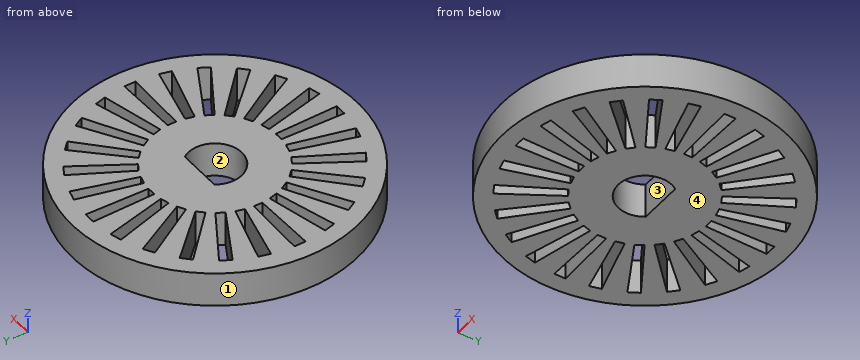
from build123d import *

# Parameters (mm, degrees)
CROQUIS1_R              = 12.84605
SALIENTE_EXTRUIR2_DEPTH = 3.1242


with BuildPart() as part:
    # Croquis1 → Saliente-Extruir2 (new body)
    with BuildSketch(Plane.XY):
        Circle(CROQUIS1_R)
        Polygon((0.508, 11.32205), (0.381, 5.73405), (-0.381, 5.73405), (-0.508, 11.32205), align=None, mode=Mode.SUBTRACT)
        Polygon((-7.646688087, -8.365108577), (-8.365108577, -7.646688087), (-4.323993322, -3.785177955), (-3.785177955, -4.323993322), align=None, mode=Mode.SUBTRACT)
        Polygon((-5.221084095, -10.059182923), (-6.100965905, -9.551182923), (-3.196980679, -4.775332967), (-2.537069321, -5.156332967), align=None, mode=Mode.SUBTRACT)
        Polygon((-2.43967185, -11.067740576), (-3.421052489, -10.804780427), (-1.852099085, -5.440056928), (-1.116063606, -5.63727704), align=None, mode=Mode.SUBTRACT)
        Polygon((-9.551182923, -6.100965905), (-10.059182923, -5.221084095), (-5.156332967, -2.537069321), (-4.775332967, -3.196980679), align=None, mode=Mode.SUBTRACT)
        Polygon((-11.32205, -0.508), (-11.32205, 0.508), (-5.73405, 0.381), (-5.73405, -0.381), align=None, mode=Mode.SUBTRACT)
        Polygon((-10.804780427, -3.421052489), (-11.067740576, -2.43967185), (-5.63727704, -1.116063606), (-5.440056928, -1.852099085), align=None, mode=Mode.SUBTRACT)
        Polygon((0.508, -11.32205), (-0.508, -11.32205), (-0.381, -5.73405), (0.381, -5.73405), align=None, mode=Mode.SUBTRACT)
        Polygon((3.421052489, -10.804780427), (2.43967185, -11.067740576), (1.116063606, -5.63727704), (1.852099085, -5.440056928), align=None, mode=Mode.SUBTRACT)
        Polygon((6.100965905, -9.551182923), (5.221084095, -10.059182923), (2.537069321, -5.156332967), (3.196980679, -4.775332967), align=None, mode=Mode.SUBTRACT)
        Polygon((8.365108577, -7.646688087), (7.646688087, -8.365108577), (3.785177955, -4.323993322), (4.323993322, -3.785177955), align=None, mode=Mode.SUBTRACT)
        Polygon((10.059182923, -5.221084095), (9.551182923, -6.100965905), (4.775332967, -3.196980679), (5.156332967, -2.537069321), align=None, mode=Mode.SUBTRACT)
        Polygon((11.067740576, -2.43967185), (10.804780427, -3.421052489), (5.440056928, -1.852099085), (5.63727704, -1.116063606), align=None, mode=Mode.SUBTRACT)
        Polygon((-11.067740576, 2.43967185), (-10.804780427, 3.421052489), (-5.440056928, 1.852099085), (-5.63727704, 1.116063606), align=None, mode=Mode.SUBTRACT)
        Polygon((-10.059182923, 5.221084095), (-9.551182923, 6.100965905), (-4.775332967, 3.196980679), (-5.156332967, 2.537069321), align=None, mode=Mode.SUBTRACT)
        with BuildLine():
            Line((-1.96747554, 1.397), (1.96747554, 1.397))
            ThreePointArc((1.96747554, 1.397), (0, -2.413), (-1.96747554, 1.397))
        make_face(mode=Mode.SUBTRACT)
        Polygon((-8.365108577, 7.646688087), (-7.646688087, 8.365108577), (-3.785177955, 4.323993322), (-4.323993322, 3.785177955), align=None, mode=Mode.SUBTRACT)
        Polygon((-6.100965905, 9.551182923), (-5.221084095, 10.059182923), (-2.537069321, 5.156332967), (-3.196980679, 4.775332967), align=None, mode=Mode.SUBTRACT)
        Polygon((-3.421052489, 10.804780427), (-2.43967185, 11.067740576), (-1.116063606, 5.63727704), (-1.852099085, 5.440056928), align=None, mode=Mode.SUBTRACT)
        Polygon((10.804780427, 3.421052489), (11.067740576, 2.43967185), (5.63727704, 1.116063606), (5.440056928, 1.852099085), align=None, mode=Mode.SUBTRACT)
        Polygon((11.32205, 0.508), (11.32205, -0.508), (5.73405, -0.381), (5.73405, 0.381), align=None, mode=Mode.SUBTRACT)
        Polygon((9.551182923, 6.100965905), (10.059182923, 5.221084095), (5.156332967, 2.537069321), (4.775332967, 3.196980679), align=None, mode=Mode.SUBTRACT)
        Polygon((2.43967185, 11.067740576), (3.421052489, 10.804780427), (1.852099085, 5.440056928), (1.116063606, 5.63727704), align=None, mode=Mode.SUBTRACT)
        Polygon((5.221084095, 10.059182923), (6.100965905, 9.551182923), (3.196980679, 4.775332967), (2.537069321, 5.156332967), align=None, mode=Mode.SUBTRACT)
        Polygon((7.646688087, 8.365108577), (8.365108577, 7.646688087), (4.323993322, 3.785177955), (3.785177955, 4.323993322), align=None, mode=Mode.SUBTRACT)
    extrude(amount=SALIENTE_EXTRUIR2_DEPTH)


solid = part.part
CAD build for the part. Positions are in the model's coordinates, mm. Face numbers are marked on the shaded views. Give positions to 0.01 mm unless a question says otherwise; leave off trailing zeros. Write each loop counter-clockwise with the first axis right and the second up, starting at its lowest first coordinate (ties: lowest second). Pieces come first, ordered by that corner, then holes. Notation, with made-up numbers: (-13.75, 31.25) -> (44.25, 31.25) arc R26 ccw to (44.25, 46.25) -> close; hole circle Ø1 at (42, -26). An arc over 180 degrees is marked (long way). Return JSON: item names as keys, results as strings.
Item 1: Two-plate mould, pull along Y, no slides. Class the marked faces 1, 2, 3 and 4: +Y half, -Y half, draft (parallel to the pull), parting line (faces both ways), or undercut.
Answer below:
{"face 1": "parting line", "face 2": "undercut", "face 3": "undercut", "face 4": "draft"}
Item 2: Drop a flat-ended pin along its axis: pin 1 (1.5 mm diameter, centred on y = -1, z = 1, fed in from -X). Give the stop position or say it passes through.
Answer below:
{"pin 1": "stops at x = -12.84"}
Item 3: Band-saw the part on A-A (x = 0). List the corners of the cut face in (y, z), then the cut area to 3 significant figures.
Answer below:
{"outline": "(-12.85, 0) -> (-11.32, 0) -> (-11.32, 3.12) -> (-12.85, 3.12) -> close; (-5.73, 0) -> (-2.41, 0) -> (-2.41, 3.12) -> (-5.73, 3.12) -> close; (1.4, 0) -> (5.73, 0) -> (5.73, 3.12) -> (1.4, 3.12) -> close; (11.32, 0) -> (12.85, 0) -> (12.85, 3.12) -> (11.32, 3.12) -> close", "area": "33.4 mm2"}
Item 4: Drill centre lines: probe 1 along Y at (x, z) = (0, 1.7); probe 2 along X at (y, z) = (-3.5, 1.3); probe 3 along Y at (x, z) = (-4, 1.9). Where is each one in solid material? Low to high.
Answer below:
{"probe 1": "y = -12.85 to -11.32, -5.73 to -2.41, 1.4 to 5.73, 11.32 to 12.85", "probe 2": "x = -12.36 to -6.92, -5.27 to 5.27, 6.92 to 12.36", "probe 3": "y = -12.21 to -7.83, -6.1 to -4.55, -4.11 to 4.11, 4.55 to 6.1, 7.83 to 12.21"}
Item 5: Band-saw the part on C-C (x = -7.25). Give the number of separate pieces and of enclosed holes in the cut face, then the cut area to 3 significant figures.
Answer below:
{"separate pieces": "8", "enclosed holes": "0", "area": "43.3 mm2"}
Item 6: Band-saw the part on B-B (y = 0). List the corners of the cut face in (x, z), then the cut area to 3 significant figures.
Answer below:
{"outline": "(-12.85, 0) -> (-11.32, 0) -> (-11.32, 3.12) -> (-12.85, 3.12) -> close; (-5.73, 0) -> (-2.41, 0) -> (-2.41, 3.12) -> (-5.73, 3.12) -> close; (2.41, 0) -> (5.73, 0) -> (5.73, 3.12) -> (2.41, 3.12) -> close; (11.32, 0) -> (12.85, 0) -> (12.85, 3.12) -> (11.32, 3.12) -> close", "area": "30.3 mm2"}
